from build123d import *

# Parameters (mm, degrees)
EXTRUDE_1_DEPTH     = 36
SKETCH_2_R          = 4.25
CUT_EXTRUDE_1_DEPTH = 5
SKETCH_3_R          = 4.25
CUT_EXTRUDE_2_DEPTH = 5
FILLET_1_R          = 4
FILLET_2_R          = 1


with BuildPart() as part:
    # Эскиз1 → Бобышка-Вытянуть1 (new body, symmetric)
    with BuildSketch(Plane.XY):
        Polygon((0, 0), (-42.426406871, 42.426406871), (-38.890872965, 45.961940777), (-15.028558569, 22.099626381), (26.253591352, 5), (60, 5), (60, 0), align=None)
        Polygon((-14.313708499, 18.556349186), (23.242640687, 3), (1.242640687, 3), align=None, mode=Mode.SUBTRACT)
    extrude(amount=EXTRUDE_1_DEPTH, both=True)

    # Эскиз2 → Вырез-Вытянуть1 (cut)
    with BuildSketch(Plane(origin=(0, 0, 0), x_dir=(0, 0, 1), z_dir=(-0.707106781, -0.707106781, 0))):
        with Locations(Location((-20, 45, 0), (0, 0, 270))):  # turned: the seam where the file's is
            Circle(SKETCH_2_R)
        with Locations(Location((20, 45, 0), (0, 0, 270))):  # turned: the seam where the file's is
            Circle(SKETCH_2_R)
    extrude(amount=-CUT_EXTRUDE_1_DEPTH, mode=Mode.SUBTRACT)

    # Эскиз3 → Вырез-Вытянуть2 (cut)
    with BuildSketch(Plane.XZ):
        with Locations(Location((45, 20, 0), (0, 0, 270))):  # turned: the seam where the file's is
            Circle(SKETCH_3_R)
        with Locations(Location((45, -20, 0), (0, 0, 270))):  # turned: the seam where the file's is
            Circle(SKETCH_3_R)
    extrude(amount=-CUT_EXTRUDE_2_DEPTH, mode=Mode.SUBTRACT)

    # Скругление1
    fillet_1_edges = [part.edges().sort_by_distance(p)[0] for p in [
        (-38.890872965, 45.961940777, 0),
        (60, 5, 0),
    ]]
    fillet(fillet_1_edges, radius=FILLET_1_R)

    # Скругление2
    fillet_2_edges = [part.edges().sort_by_distance(p)[0] for p in [
        (-14.313708499, 18.556349186, 0),
        (1.242640687, 3, 0),
        (23.242640687, 3, 0),
    ]]
    fillet(fillet_2_edges, radius=FILLET_2_R)


solid = part.part
Can you work these out from the model? Positions are in its coordinate system, mm. A direction names the side the tool comes from. Give positions to 0.01 mm unless a question says otherwise; leave off trailing zeros. Loops run counter-clockwise (first coordinate to the right, second up) from the corner with the lowest first, then second, coordinate; pieces in that order, holes last. Notation, with made-up numbers: (67.5, 47) - (88.5, 47) arc R20 cw to (88.5, 82) - close; hole circle Ø4 at (-14.5, 12). An arc over 180 degrees is marked (long way). One line per item, written item: value.
(1) If we section it at C-C, the plane z = 30.5: List the corners of the cut face in (x, y) for me.
Verdict:
outline: (-42.43, 42.43) - (0, 0) - (60, 0) - (60, 1) arc R4 ccw to (56, 5) - (26.25, 5) - (-15.03, 22.1) - (-36.06, 43.13) arc R4 ccw to (-41.72, 43.13) - close; hole (-10.76, 15) - (0.95, 3.29) arc R1 ccw to (1.66, 3) - (18.22, 3) arc R1 ccw to (18.6, 4.92) - (-9.67, 16.63) arc R1 ccw to start
(2) If we mould it in two halves opening along Y, with no side actions, what happens to faces 1 (the face through (40.85, 2.46, 20.92)), 2 (the face through (41, 5, 1)), 3 (the face through (-30.73, 34.21, -24.15))? For each: released by +Y, released by -Y, zero draft, split by the parting line, or undercut.
Verdict:
face 1: zero draft
face 2: released by +Y
face 3: undercut
(3) If we section it at B-B, the plane z = -20: List the corners of the cut face in (x, y) for me (3 decimals).
Verdict:
outline: (-42.426, 42.426) - (-34.825, 34.825) - (-31.289, 38.361) - (-36.062, 43.134) arc R4 ccw to (-41.719, 43.134) - close; (-28.815, 28.815) - (0, 0) - (40.75, 0) - (40.75, 5) - (26.254, 5) - (-15.029, 22.1) - (-25.279, 32.35) - close; (49.25, 0) - (60, 0) - (60, 1) arc R4 ccw to (56, 5) - (49.25, 5) - close; hole (-10.759, 15.001) - (0.95, 3.293) arc R1 ccw to (1.657, 3) - (18.215, 3) arc R1 ccw to (18.598, 4.924) - (-9.669, 16.632) arc R1 ccw to start
(4) If we section it at D-D, the plane x = -3: List the corners of the cut face in (y, z) for me.
Verdict:
outline: (3, -36) - (7.24, -36) - (7.24, 36) - (3, 36) - close; (13.87, -36) - (17.12, -36) - (17.12, 36) - (13.87, 36) - close
(5) If we section it at A-A, the plane x = 45: List the corners of the cut face in (y, z) for me.
Verdict:
outline: (0, -36) - (5, -36) - (5, -24.25) - (0, -24.25) - close; (0, -15.75) - (5, -15.75) - (5, 15.75) - (0, 15.75) - close; (0, 24.25) - (5, 24.25) - (5, 36) - (0, 36) - close
(6) On a 3-axis mill with a long thin cutter (end or side, diameter ignored), from which of +Z, -Z, +X, -X, +Y, -Y can I reach the whole of each face in a straight line? I mean faces 4 (the face through (10, 3, 1)), 5 (the face through (5.32, 13.67, 0.5)). Say none if no direction works.
Verdict:
face 4: +Z, -Z
face 5: +Z, -Z, +X, +Y
(7) I need wall thicknesses on line 1 along Y through (x, z) = (8.5, -16); line 2 along Y through (x, z) = (40.5, 1); line 3 along Y through (x, z) = (8, -16). Which ranges of each line are inside material? Lowest first, please.
Verdict:
line 1: 0 to 3, 9.11 to 12.35
line 2: 0 to 5
line 3: 0 to 3, 9.31 to 12.56
(8) I'm going to push flat-ended pins straight in: pin 1 (10 mm diameter, centred on x = 28, z = 27, fed in from +Y); pin 2 (5 mm diameter, centred on x = 12.5, z = -1.5, fed in from +Y); pin 3 (10 mm diameter, centred on x = 36, z = -18.5, fed in from +Y); pin 4 (7 mm diameter, centred on x = 45, z = 20, fed in from -Y). Where does each tip first touch, or does it pass through?
Verdict:
pin 1: y = 6.35
pin 2: y = 11.73
pin 3: y = 5
pin 4: through
